```python
from build123d import *

# Parameters (mm, degrees)
ESQUISSE1_R             = 50
BOSS_EXTRU_1_DEPTH      = 20
ESQUISSE2_R             = 50
ESQUISSE2_R_2           = 48
BOSS_EXTRU_2_DEPTH      = 10
ESQUISSE3_OUTSIDE_W     = 713.342
ESQUISSE3_OUTSIDE_H     = 263.342
ENL_V_MAT_EXTRU_1_DEPTH = 21


with BuildPart() as part:
    # Esquisse1 → Boss.-Extru.1 (new body)
    with BuildSketch(Plane.XY):
        with BuildLine():
            Line((0, -70), (-450, -70))
            ThreePointArc((-450, -70), (-520, 0), (-450, 70))
            Line((-450, 70), (0, 70))
            ThreePointArc((0, 70), (70, 0), (0, -70))
        make_face()
        Circle(ESQUISSE1_R, mode=Mode.SUBTRACT)
    extrude(amount=BOSS_EXTRU_1_DEPTH)

    # Esquisse2 → Boss.-Extru.2 (add)
    with BuildSketch(Plane(origin=(0, 0, 0), x_dir=(-1, 0, 0), z_dir=(0, 0, -1))):
        Circle(ESQUISSE2_R)
        Circle(ESQUISSE2_R_2, mode=Mode.SUBTRACT)
    extrude(amount=-BOSS_EXTRU_2_DEPTH)

    # Esquisse3 outside → Enlèv. mat.-Extru.1 (cut, through all)
    with BuildSketch(Plane(origin=(0, 0, 0), x_dir=(-1, 0, 0), z_dir=(0, 0, -1))):
        with Locations((225, 0)):
            Rectangle(ESQUISSE3_OUTSIDE_W, ESQUISSE3_OUTSIDE_H)
        with BuildLine():
            Line((450, -50), (48.989794856, -50))
            ThreePointArc((48.989794856, -50), (-70, 0), (48.989794856, 50))
            Line((48.989794856, 50), (450, 50))
            ThreePointArc((450, 50), (500, 0), (450, -50))
        make_face(mode=Mode.SUBTRACT)
    extrude(amount=-ENL_V_MAT_EXTRU_1_DEPTH, mode=Mode.SUBTRACT)


solid = part.part
```
Model file for the job. Use its own axes, mm. A direction names the side the tool comes from. Round coordinates to 2 decimals unless told otherwise and drop trailing zeros. Write each loop counter-clockwise with the first axis right and the second up, starting at its lowest first coordinate (ties: lowest second). Pieces come first, ordered by that corner, then holes. Notation, with made-up numbers: (55, 31.25) - (86, 31.25) arc R24 cw to (86, 69.25) - close; hole circle Ø5 at (64, -20). An arc over 180 degrees is marked (long way). Use CSV: the item, a comma, the result in double quotes. Start each with the question number.
Item 1: Band-saw the part on D-D (x = -270.5). Write the cut outline in (y, z).
Item 2: Band-saw the part on A-A (y = 0). Write the cut outline in (x, z), and give its area (3 significant figures).
Item 3: Band-saw the part on B-B (z = 4.75). Write the cut outline in (x, y).
Item 4: Tool access for faces 4 (the face through (-247, 50, 10)), 5 (the face through (-211, 1, 20)), 6 (the face through (47.69, 15.02, 14.93)), 7 (the face through (-252, -50, 10)), 8 (the face through (47.954, 2.11, 4.93)): list every direction of +Z, -Z, +X, -X, +Y, -Y with a clear straight run to the whole face (end or side of a thin tool).
Item 5: Drill centre lines: L1, parallel to X at y = 32.5, z = 7.5; L2, parallel to Y at x = -306, z = 17.5; L3, parallel to X at y = -10.5, z = 1.75. Where is each one in solid material? Low to high. Write a range as [from, to].
Item 6: Band-saw the part on C-C (y = 22.5). Write the cut outline in (x, z), and give its area (3 significant figures).
Item 7: Two-plate mould, pull along X, no slides. Class faces 1 (the face through (19, 45, 10)), 2 (the face through (-499.988, 1.099, 9.86)), 3 (the face through (-211, 1, 0)): released by +X, released by -X, zero draft, split by the parting line, or undercut.
Item 8: Pin check, flat tips, straight feed: P1, Ø3, axis at x = -426, z = 11, coming from the -Y side; P2, Ø3, axis at y = -46, z = 7, coming from the -X side; P3, Ø12, axis at x = -370, z = 15, coming from the +Y side. Stop position of each tip, or through.
Checked values:
1,outline,"(-50, 0) - (50, 0) - (50, 20) - (-50, 20) - close"
2,outline,"(-500, 0) - (-48, 0) - (-48, 10) - (-50, 10) - (-50, 20) - (-500, 20) - close; (48, 0) - (70, 0) - (70, 20) - (50, 20) - (50, 10) - (48, 10) - close"
2,area,"9,440 mm²"
3,outline,"(-450, -50) - (-48.99, -50) arc R70 ccw (long way) to (-48.99, 50) - (-450, 50) arc R50 ccw to start; hole circle Ø96 at (0, 0)"
4,face 4,"+Z, -Z, -X, +Y"
4,face 5,"+Z, +X, -X, +Y, -Y"
4,face 6,"+Z"
4,face 7,"+Z, -Z, -X, -Y"
4,face 8,"+Z, -Z"
5,L1,"x = [-488, -35.32], [35.32, 62]"
5,L2,"y = [-50, 50]"
5,L3,"x = [-498.89, -46.84], [46.84, 69.21]"
6,outline,"(-494.65, 0) - (-42.4, 0) - (-42.4, 10) - (-44.65, 10) - (-44.65, 20) - (-494.65, 20) - close; (42.4, 0) - (66.29, 0) - (66.29, 20) - (44.65, 20) - (44.65, 10) - (42.4, 10) - close"
6,area,"9,480 mm²"
7,face 1,"undercut"
7,face 2,"released by -X"
7,face 3,"zero draft"
8,P1,"stops at y = -50"
8,P2,"stops at x = -472.8"
8,P3,"stops at y = 50"
